Design review of the part built by this model. Coordinates are the model's own, in mm. Face numbers are marked on the shaded views. A direction names the side the tool comes from. Round coordinates to 2 decimals unless told otherwise and drop trailing zeros. Loops run counter-clockwise (first coordinate to the right, second up) from the corner with the lowest first, then second, coordinate; pieces in that order, holes last. Notation, with made-up numbers: (54, 85) -> (110, 85) arc R21 ccw to (110, 104) -> close; hole circle Ø9 at (-1, -31). An arc over 180 degrees is marked (long way). Answer as CSV lines item,"result". Start each with the question number.
```python
from build123d import *

# Parameters (mm, degrees)
CSK_FOR_M12_HEX_SOCKET_COUNTERSUNK_CAP_S_D           = 14
CSK_FOR_M12_HEX_SOCKET_COUNTERSUNK_CAP_S_DEPTH       = 27
CSK_FOR_M12_HEX_SOCKET_COUNTERSUNK_CAP_S_CSINK_D     = 26
CSK_FOR_M12_HEX_SOCKET_COUNTERSUNK_CAP_S_CSINK_ANGLE = 90
CSK_FOR_M12_HEX_SOCKET_COUNTERSUNK_CAP_S_TIP         = 4.206024333
CSK_FOR_M6_HEX_SOCKET_COUNTERSUNK_CAP_SC_D           = 6.5
CSK_FOR_M6_HEX_SOCKET_COUNTERSUNK_CAP_SC_CSINK_D     = 7.5
CSK_FOR_M6_HEX_SOCKET_COUNTERSUNK_CAP_SC_CSINK_ANGLE = 90
CIRPATTERN1_COUNT                                    = 6


with BuildPart() as part:
    # Sketch1 → Revolve1 (revolve)
    with BuildSketch(Plane.XY):
        Polygon((-20.025316456, 0), (-20.025316456, 35), (-15.025316456, 35), (-15.025316456, 47.5), (-10.025316456, 47.5), (-10.025316456, 14), (7.974683544, 14), (7.974683544, 0), align=None)
    revolve(axis=Axis((-20.025316456, 0, 0), (1, 0, 0)))

    # CSK for M12 Hex Socket Countersunk Cap Screw1
    with Locations(Plane.ZY.offset(20.025316456)):
        with Locations((0, 0)):
            CounterSinkHole(CSK_FOR_M12_HEX_SOCKET_COUNTERSUNK_CAP_S_D / 2, CSK_FOR_M12_HEX_SOCKET_COUNTERSUNK_CAP_S_CSINK_D / 2, depth=CSK_FOR_M12_HEX_SOCKET_COUNTERSUNK_CAP_S_DEPTH, counter_sink_angle=CSK_FOR_M12_HEX_SOCKET_COUNTERSUNK_CAP_S_CSINK_ANGLE)
            with Locations((0, 0, -(CSK_FOR_M12_HEX_SOCKET_COUNTERSUNK_CAP_S_DEPTH + CSK_FOR_M12_HEX_SOCKET_COUNTERSUNK_CAP_S_TIP / 2))):  # 118° drill point
                Cone(0, CSK_FOR_M12_HEX_SOCKET_COUNTERSUNK_CAP_S_D / 2, CSK_FOR_M12_HEX_SOCKET_COUNTERSUNK_CAP_S_TIP, mode=Mode.SUBTRACT)

    # CSK for M6 Hex Socket Countersunk Cap Screw1 (through all)
    with Locations(Plane.ZY.offset(20.025316456)):
        with Locations((0, 40)):
            csk_for_m6_hex_socket_countersunk_cap_sc = CounterSinkHole(CSK_FOR_M6_HEX_SOCKET_COUNTERSUNK_CAP_SC_D / 2, CSK_FOR_M6_HEX_SOCKET_COUNTERSUNK_CAP_SC_CSINK_D / 2, counter_sink_angle=CSK_FOR_M6_HEX_SOCKET_COUNTERSUNK_CAP_SC_CSINK_ANGLE)

    # CirPattern1: CSK for M6 Hex Socket Countersunk Cap Screw1 ×6 about axis
    cirpattern1_axis = Axis((0, 0, 0), (1, 0, 0))
    for i in range(1, CIRPATTERN1_COUNT):
        add(csk_for_m6_hex_socket_countersunk_cap_sc.rotate(cirpattern1_axis, i * 360 / CIRPATTERN1_COUNT), mode=Mode.SUBTRACT)


solid = part.part
```
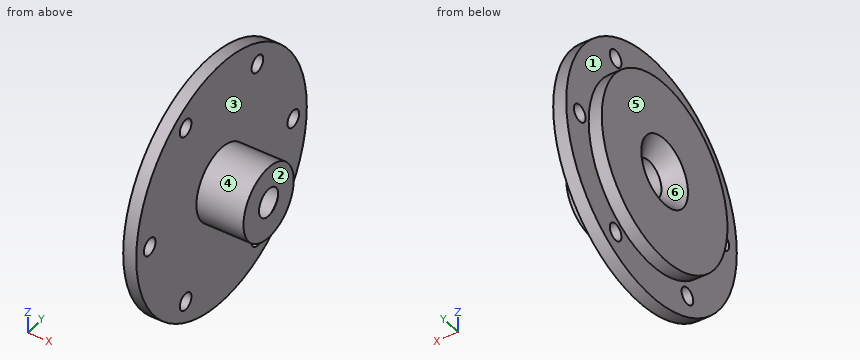
Q1. Mouldability with a two-part tool opening along Y and no side actions: class the marked faces 4, 5 and 6 as pulls with the +Y half, pulls with the -Y half, needs draft (parallel to the pull), parting line crosses it, or undercut.
Q2. To check wall thickness, follow probe 1 along X at (y, z) = (23.5, -19.5); probe 2 along X at (y, z) = (29.5, -29); probe 3 along Z at (x, y) = (-12.75, -22.5). State the ranges of each line that lie inside material, in increasing order. Write a range as from..to.
Q3. Add section A-A, the plane z = 0. Give the boundary of the cut face in (x, y).
Q4. For pin 1 Ø6 at (x, z) = (-16, 32.5) entering from +Y; pin 2 Ø6 at (y, z) = (-30, -11.5) entering from +X; pin 3 Ø4 at (x, y) = (-15, -21) entering from -Z, all flat-tipped, find the tip position at first contact; note any pin that passes through.
Q5. Machinability: for the marked faces 1, 2 and 3, which of the approach directions +Z, -Z, +X, -X, +Y, -Y give a long, thin tool a straight path to every point of the face, cutting with its end or side? Answer none if there is none.
Q6. Add section D-D, the plane x = 4. Give the boundary of the cut face in (y, z).
Q7. Add section C-C, the plane y = 0. Give the boundary of the cut face in (x, z), and give its area (3 significant figures).
Q8. Add section B-B, the plane y = 20. Give the boundary of the cut face in (x, z), and give its area (3 significant figures).
Worked answers:
1,face 4,"parting line crosses it"
1,face 5,"needs draft"
1,face 6,"undercut"
2,probe 1,"x = -20.03..-10.03"
2,probe 2,"x = -15.03..-10.03"
2,probe 3,"z = -41.83..-36.72, -32.56..32.56, 36.72..41.83"
3,outline,"(-20.03, -35) -> (-15.03, -35) -> (-15.03, -36.75) -> (-10.03, -36.75) -> (-10.03, -14) -> (7.97, -14) -> (7.97, -5.34) -> (6.97, -7) -> (-14.03, -7) -> (-20.03, -13) -> close; (-20.03, 13) -> (-14.03, 7) -> (6.97, 7) -> (7.97, 5.34) -> (7.97, 14) -> (-10.03, 14) -> (-10.03, 36.75) -> (-15.03, 36.75) -> (-15.03, 35) -> (-20.03, 35) -> close; (-15.03, -47.5) -> (-10.03, -47.5) -> (-10.03, -43.25) -> (-15.03, -43.25) -> close; (-15.03, 43.25) -> (-10.03, 43.25) -> (-10.03, 47.5) -> (-15.03, 47.5) -> close"
4,pin 1,"stops at y = 37.1"
4,pin 2,"stops at x = -10.03"
4,pin 3,"stops at z = -43.53"
5,face 1,"-X"
5,face 2,"+Z, -Z, +X, +Y, -Y"
5,face 3,"+X"
6,outline,"circle Ø28 at (0, 0); hole circle Ø14 at (0, 0)"
7,outline,"(-20.03, -35) -> (-15.03, -35) -> (-15.03, -47.5) -> (-10.03, -47.5) -> (-10.03, -14) -> (7.97, -14) -> (7.97, -5.34) -> (6.97, -7) -> (-14.03, -7) -> (-20.03, -13) -> close; (-20.03, 13) -> (-14.03, 7) -> (6.97, 7) -> (7.97, 5.34) -> (7.97, 14) -> (-10.03, 14) -> (-10.03, 47.5) -> (-15.03, 47.5) -> (-15.03, 35) -> (-20.03, 35) -> close"
7,area,"903 mm^2"
8,outline,"(-20.03, -28.72) -> (-15.03, -28.72) -> (-15.03, -31.39) -> (-10.03, -31.39) -> (-10.03, 31.39) -> (-15.03, 31.39) -> (-15.03, 28.72) -> (-20.03, 28.72) -> close; (-15.03, -43.08) -> (-10.03, -43.08) -> (-10.03, -37.89) -> (-15.03, -37.89) -> close; (-15.03, 37.89) -> (-10.03, 37.89) -> (-10.03, 43.08) -> (-15.03, 43.08) -> close"
8,area,"653 mm^2"
